from build123d import *

# Parameters (mm, degrees)
SKETCH2_R           = 42.5
BOSS_EXTRUDE1_DEPTH = 160
SKETCH3_R           = 15
BOSS_EXTRUDE2_DEPTH = 60
FILLET1_R           = 20
FILLET2_R           = 10
BOSS_EXTRUDE3_START = 1
SKETCH4_R           = 16
BOSS_EXTRUDE3_DEPTH = 20
BOSS_EXTRUDE4_START = -10
SKETCH5_R           = 43
BOSS_EXTRUDE4_DEPTH = 100


with BuildPart() as part:
    # Sketch2 → Boss-Extrude1 (new body)
    with BuildSketch(Plane(origin=(0, 0, 0), x_dir=(1, 0, 0), z_dir=(0, 1, 0))):
        with Locations(Location((0, 0, 0), (0, 0, 270))):
            Circle(SKETCH2_R)
    extrude(amount=BOSS_EXTRUDE1_DEPTH)

    # Sketch3 → Boss-Extrude2 (add)
    with BuildSketch(Plane(origin=(0, 160, 0), x_dir=(1, 0, 0), z_dir=(0, 1, 0))):
        with Locations(Location((0, 0, 0), (0, 0, 270))):
            Circle(SKETCH3_R)
    extrude(amount=BOSS_EXTRUDE2_DEPTH)

    # Fillet1
    fillet1_edges = [part.edges().sort_by_distance(p)[0] for p in [
        (0, 160, -15),
    ]]
    fillet(fillet1_edges, radius=FILLET1_R)

    # Fillet2
    fillet2_edges = [part.edges().sort_by_distance(p)[0] for p in [
        (0, 160, -42.5),
    ]]
    fillet(fillet2_edges, radius=FILLET2_R)

    # Sketch4 → Boss-Extrude3 (add)
    with BuildSketch(Plane(origin=(0, 220, 0), x_dir=(1, 0, 0), z_dir=(0, 1, 0)).offset(BOSS_EXTRUDE3_START)):
        with Locations(Location((0, 0, 0), (0, 0, 270))):
            Circle(SKETCH4_R)
    extrude(amount=-BOSS_EXTRUDE3_DEPTH)

    # Sketch5 → Boss-Extrude4 (add)
    with BuildSketch(Plane.XZ.offset(BOSS_EXTRUDE4_START)):
        with Locations(Location((0, 0, 0), (0, 0, 270))):
            Circle(SKETCH5_R)
    extrude(amount=-BOSS_EXTRUDE4_DEPTH)


solid = part.part
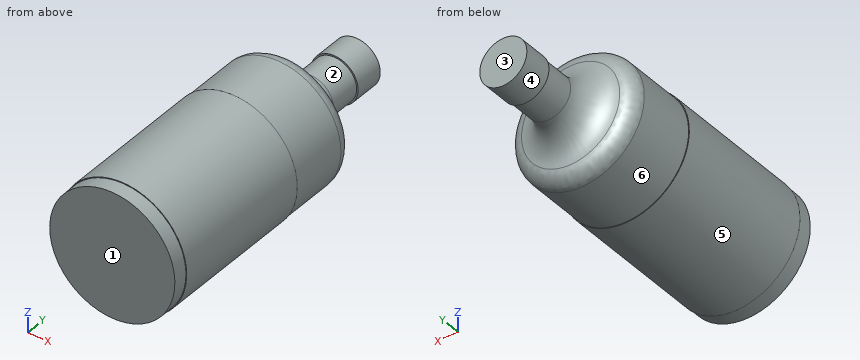
Build history of the part. All positions in model axes, mm. Face numbers are marked on the shaded views. A direction names the side the tool comes from. Round coordinates to 2 decimals unless told otherwise and drop trailing zeros. Loops run counter-clockwise (first coordinate to the right, second up) from the corner with the lowest first, then second, coordinate; pieces in that order, holes last. Notation, with made-up numbers: (36, -15) -> (45, -15) arc R25 cw to (45, 23) -> close; hole circle Ø7 at (53, 8). An arc over 180 degrees is marked (long way). Use CSV: the item, a comma, the result in double quotes. Start each with the question number.
Q1. Drill centre lines: L1, parallel to X at y = 56.5, z = -6.5; L2, parallel to Z at x = -27, y = 24; L3, parallel to Z at x = -1, y = 195. Where is each one in solid material? Low to high.
Q2. Which spindle directions (+Z, -Z, +X, -X, +Y, -Y) get a long thin tool onto all of the face, cutting with end or side? Do the marked faces 5 and 6. Say none if no direction does.
Q3. Saw through at A-A on y = 65. Give the cut face in (x, z), and give its area (3 significant figures).
Q4. Flat gauge pins, fed straight in: pin 1 Ø1 at (x, z) = (3, -34) entering from +Y; pin 2 Ø1.5 at (x, y) = (-10.5, 113.5) entering from -Z; pin 3 Ø6 at (y, z) = (157.5, 3) entering from +X; pin 4 Ø3 at (x, z) = (-4.5, -8.5) entering from -Y. Where does each tip first touch, or does it go through?
Q5. Mould opens along Y. For the marked faces 1, 2, 3 and 4 say: +Y half, -Y half, draft (parallel to the pull), parting line (faces both ways), or undercut.
Q6. Saw through at B-B on y = 119. Give the cut face in (x, z).
Solutions:
1,L1,"x = -42.51 to 42.51"
1,L2,"z = -33.47 to 33.47"
1,L3,"z = -14.97 to 14.97"
2,face 5,"+Y, -Y"
2,face 6,"+Y"
3,outline,"circle Ø86 at (0, 0)"
3,area,"5,810 mm^2"
4,pin 1,"stops at y = 160.04"
4,pin 2,"stops at z = -41.37"
4,pin 3,"stops at x = 41.39"
4,pin 4,"stops at y = 0"
5,face 1,"-Y half"
5,face 2,"undercut"
5,face 3,"+Y half"
5,face 4,"draft"
6,outline,"circle Ø85 at (0, 0)"
